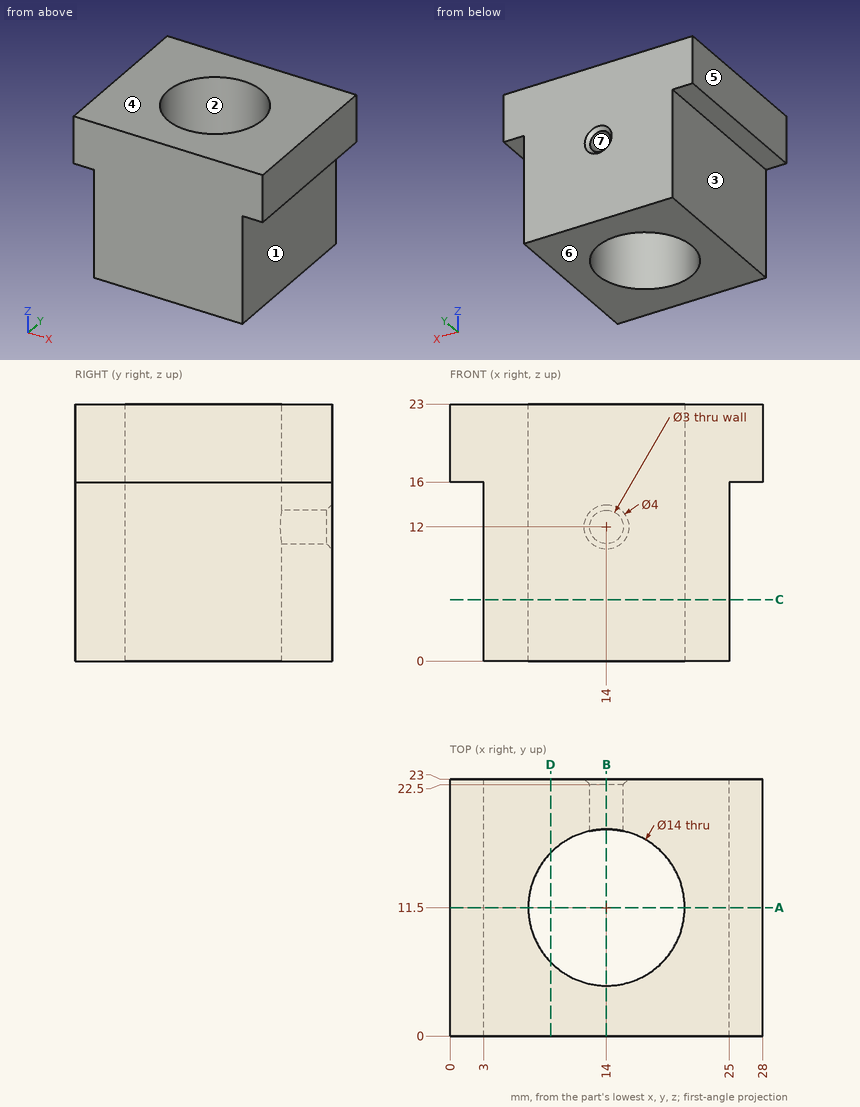
Part print with two shaded views. Sizes in mm from the minimum x, y, z corner. A direction names the side the tool comes from. Round coordinates to 2 decimals unless told otherwise and drop trailing zeros. Order: outer loops, then holes, each group sorted by start corner. A loop starts at its lowest first (then second) coordinate and runs counter-clockwise, first axis right, second up.
(1) Band-saw the part on C-C (z = 5.5). List the corners of the cut face in (x, y), then the cut area to 3 significant figures.
(2) Pull direction Z, two halves, no side cores. Call the marked faces 4, 5, 6 and 7: released by +Z, released by -Z, zero draft, split by the parting line, or undercut.
(3) Band-saw the part on D-D (x = 9). List the corners of the cut face in (y, z).
(4) Band-saw the part on A-A (y = 11.5). List the corners of the cut face in (x, z), then the cut area to 3 significant figures.
(5) Drill centre lines: line 1 (Z direction, x = 14, y = 20.35); line 2 (Y direction, x = 14, z = 9.75); line 3 (X direction, y = 18.75, z = 8.25). Where is each one in solid material? Low to high.
(6) Pin check, flat tip, straight feed: pin 1 (13 mm diameter, centred on y = 10.5, z = 6, fed in from +X). Stop position of the tip, or through.
(7) 3-axis set-ups, long thin cutter, end or side, ignore diameter. For the marked faces 1, 2 and 3: which of +Z, -Z, +X, -X, +Y, -Y reach the whole face in a straight line?
(8) Band-saw the part on B-B (x = 14). List the corners of the cut face in (y, z), then the cut area to 3 significant figures.
Verdict:
1. outline: (3, 0) - (25, 0) - (25, 23) - (3, 23) - close; hole circle Ø14 at (14, 11.5)
1. area: 352 mm2
2. face 4: released by +Z
2. face 5: zero draft
2. face 6: released by -Z
2. face 7: undercut
3. outline: (0, 0) - (6.6, 0) - (6.6, 23) - (0, 23) - close; (16.4, 0) - (23, 0) - (23, 23) - (16.4, 23) - close
4. outline: (0, 16) - (3, 16) - (3, 0) - (7, 0) - (7, 23) - (0, 23) - close; (21, 0) - (25, 0) - (25, 16) - (28, 16) - (28, 23) - (21, 23) - close
4. area: 226 mm2
5. line 1: z = 0 to 10.5, 13.5 to 23
5. line 2: y = 0 to 4.5, 18.5 to 23
5. line 3: x = 3 to 25
6. pin 1: stops at x = 25
7. face 1: -Z, +X, +Y, -Y
7. face 2: +Z, -Z
7. face 3: -Z, -X, +Y, -Y
8. outline: (0, 0) - (4.5, 0) - (4.5, 23) - (0, 23) - close; (18.5, 0) - (23, 0) - (23, 10) - (22.5, 10.5) - (18.5, 10.5) - close; (18.5, 13.5) - (22.5, 13.5) - (23, 14) - (23, 23) - (18.5, 23) - close
8. area: 193 mm2
